The model under review builds one solid part; all positions refer to its coordinate system, in mm. Coordinates: 2 decimals unless noted, no trailing zeros. Write each loop counter-clockwise with the first axis right and the second up, starting at its lowest first coordinate (ties: lowest second). Pieces come first, ordered by that corner, then holes. Notation, with made-up numbers: M -26,5 L 32,5 A23 cw 32,22 Z; hole C 41.25,3 d9. An arc over 180 degrees is marked long. Answer as a JSON object with one key per item and string values.
```python
from build123d import *

# Parameters (mm, degrees)
SKETCH1_W           = 152.4
SKETCH1_H           = 88.9
BOSS_EXTRUDE1_DEPTH = 152.4
SKETCH2_R           = 13.843
CUT_EXTRUDE1_DEPTH  = 234.141008834
SKETCH3_R           = 5.1562
CUT_EXTRUDE2_DEPTH  = 234.141008834


with BuildPart() as part:
    # Sketch1 → Boss-Extrude1 (new body)
    with BuildSketch(Plane.XY):
        with Locations((76.2, 44.45)):
            Rectangle(SKETCH1_W, SKETCH1_H)
    extrude(amount=BOSS_EXTRUDE1_DEPTH)

    # Sketch2 → Cut-Extrude1 (cut, through all)
    with BuildSketch(Plane.XY):
        with Locations((76.2, 44.45)):
            Circle(SKETCH2_R)
    extrude(amount=CUT_EXTRUDE1_DEPTH, mode=Mode.SUBTRACT)

    # Sketch3 → Cut-Extrude2 (cut, through all)
    with BuildSketch(Plane.XY):
        with Locations((12.7, 44.45)):
            Circle(SKETCH3_R)
        with Locations((139.7, 44.45)):
            Circle(SKETCH3_R)
    extrude(amount=CUT_EXTRUDE2_DEPTH, mode=Mode.SUBTRACT)


solid = part.part
```
(1) For pin 1 Ø12 at (y, z) = (71, 18.5) entering from -X, flat-tipped, find the tip position at first contact; note if it passes through.
Results list:
{"pin 1": "x = 0"}
(2) Add section A-A on x = 76.2. Give the boundary of the cut face in (y, z).
Results list:
{"outline": "M 0,0 L 30.61,0 L 30.61,152.4 L 0,152.4 Z; M 58.29,0 L 88.9,0 L 88.9,152.4 L 58.29,152.4 Z"}
(3) Add section D-D on y = 34.5. Give the boundary of the cut face in (x, z), and give its area (3 significant figures).
Results list:
{"outline": "M 0,0 L 66.58,0 L 66.58,152.4 L 0,152.4 Z; M 85.82,0 L 152.4,0 L 152.4,152.4 L 85.82,152.4 Z", "area": "20,300 mm²"}
(4) Add section C-C on y = 44.45. Give the boundary of the cut face in (x, z).
Results list:
{"outline": "M 0,0 L 7.54,0 L 7.54,152.4 L 0,152.4 Z; M 17.86,0 L 62.36,0 L 62.36,152.4 L 17.86,152.4 Z; M 90.04,0 L 134.54,0 L 134.54,152.4 L 90.04,152.4 Z; M 144.86,0 L 152.4,0 L 152.4,152.4 L 144.86,152.4 Z"}
(5) Add section B-B on z = 96.5. Give the boundary of the cut face in (x, y).
Results list:
{"outline": "M 0,0 L 152.4,0 L 152.4,88.9 L 0,88.9 Z; hole C 12.7,44.45 d10.31; hole C 76.2,44.45 d27.69; hole C 139.7,44.45 d10.31"}
(6) Draft analysis for pull direction Y (two halves, no side actions). For faces 1 (the face through (75, 88.9, 75)), 2 (the face through (0, 44, 75)), 3 (the face through (11.582, 39.416, 75.133)), state which applies: released by +Y, released by -Y, zero draft, split by the parting line, or undercut.
Results list:
{"face 1": "released by +Y", "face 2": "zero draft", "face 3": "undercut"}
(7) Wall thickness on line 1 along X through (y, z) = (44.45, 90.5); line 2 along X through (y, z) = (44, 106); line 3 along Y through (x, z) = (76, 107): over which ranges is each line inside the solid? List them lowest first. Write a range as from..to.
Results list:
{"line 1": "0..7.54, 17.86..62.36, 90.04..134.54, 144.86..152.4", "line 2": "0..7.56, 17.84..62.36, 90.04..134.56, 144.84..152.4", "line 3": "0..30.61, 58.29..88.9"}
